Geometry check sheet. Reference: drawing and pictorial views, mm from the part's lowest x, y, z. Round coordinates to 2 decimals unless told otherwise and drop trailing zeros. Write each loop counter-clockwise with the first axis right and the second up, starting at its lowest first coordinate (ties: lowest second). Pieces come first, ordered by that corner, then holes. Notation, with made-up numbers: (41, 82.5) - (75, 82.5) arc R25 ccw to (75, 106.5) - close; hole circle Ø9 at (62.25, -22). An arc over 180 degrees is marked (long way). Return JSON: item names as keys, results as strings.
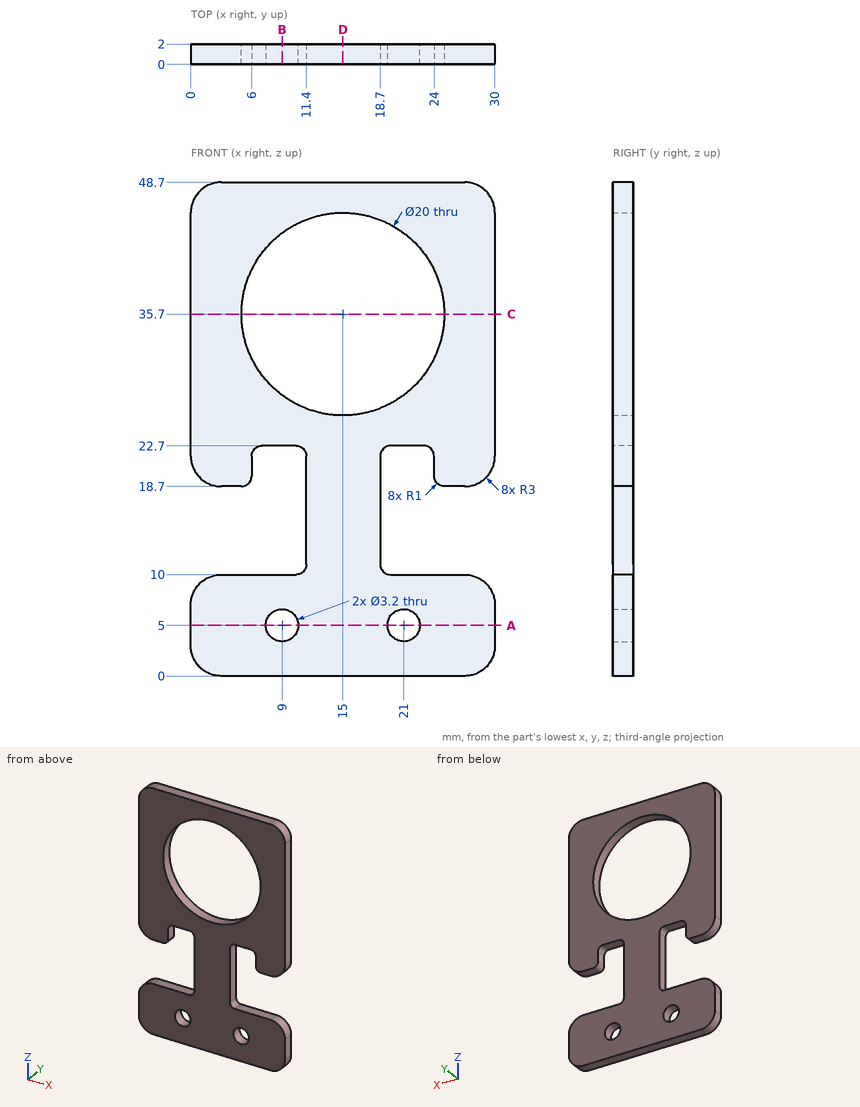
(1) Section check B-B, the plane x = 9. Enter the section's corners in (y, z), plus the area to 3 significant figures.
Response values:
{"outline": "(0, 0) - (2, 0) - (2, 3.4) - (0, 3.4) - close; (0, 6.6) - (2, 6.6) - (2, 10) - (0, 10) - close; (0, 22.7) - (2, 22.7) - (2, 27.7) - (0, 27.7) - close; (0, 43.7) - (2, 43.7) - (2, 48.7) - (0, 48.7) - close", "area": "33.6 mm^2"}
(2) Section check C-C, the plane z = 35.7. Enter the section's corners in (x, y).
Response values:
{"outline": "(0, 0) - (5, 0) - (5, 2) - (0, 2) - close; (25, 0) - (30, 0) - (30, 2) - (25, 2) - close"}
(3) Section check A-A, the plane z = 5. Enter the section's corners in (x, y).
Response values:
{"outline": "(0, 0) - (7.4, 0) - (7.4, 2) - (0, 2) - close; (10.6, 0) - (19.4, 0) - (19.4, 2) - (10.6, 2) - close; (22.6, 0) - (30, 0) - (30, 2) - (22.6, 2) - close"}
(4) Gauge pin test, flat ends, axial feed: pin 1 (3 mm diameter, centred on x = 9, z = 5, fed in from -Y); pin 2 (1 mm diameter, centred on y = 1, z = 20.5, fed in from -X). Record the tip position at first contact, or that the pin passes through.
Response values:
{"pin 1": "passes through", "pin 2": "stops at x = 0.08"}
(5) Material ranges on line 1 along X through (y, z) = (0.8, 35.7); line 2 along Z through (x, y) = (3, 1.75); line 3 along Z through (x, y) = (9, 1.4), recorded low to high. Write a range as [from, to].
Response values:
{"line 1": "x = [0, 5], [25, 30]", "line 2": "z = [0, 10], [18.7, 48.7]", "line 3": "z = [0, 3.4], [6.6, 10], [22.7, 27.7], [43.7, 48.7]"}
(6) Section check D-D, the plane x = 15. Enter the section's corners in (y, z), plus the area to 3 significant figures.
Response values:
{"outline": "(0, 0) - (2, 0) - (2, 25.7) - (0, 25.7) - close; (0, 45.7) - (2, 45.7) - (2, 48.7) - (0, 48.7) - close", "area": "57.4 mm^2"}
